```python
from build123d import *

# Parameters (mm, degrees)
SKETCH_1_W          = 120
SKETCH_1_H          = 94
SKETCH_1_R          = 37
EXTRUDE_2_DEPTH     = 4
SKETCH_2_W          = 15
SKETCH_2_H          = 74
CUT_EXTRUDE_1_DEPTH = 10
FILLET_1_R          = 8
FILLET_2_R          = 8
SKETCH_5_R          = 1.6
CUT_EXTRUDE_2_DEPTH = 10
SKETCH_6_W          = 10
SKETCH_6_H          = 43
EXTRUDE_3_DEPTH     = 4
FILLET_3_R          = 3.8
FILLET_4_R          = 15
SKETCH_7_R          = 1.6
CUT_EXTRUDE_3_DEPTH = 109.240473022
CUT_EXTRUDE_4_DEPTH = 10
FILLET_5_DEPTH      = 4
FILLET_6_R          = 5
MIRROR_1_DEPTH      = 4
SKETCH_10_R         = 1.6
CUT_EXTRUDE_6_DEPTH = 109.240473022


with BuildPart() as part:
    # 草图1 → 凸台-拉伸2 (new body)
    with BuildSketch(Plane(origin=(0, 0, 0), x_dir=(1, 0, 0), z_dir=(0, 1, 0))):
        Rectangle(SKETCH_1_W, SKETCH_1_H)
        with Locations(Location((0, 0, 0), (0, 0, 270))):
            Circle(SKETCH_1_R, mode=Mode.SUBTRACT)
    extrude(amount=EXTRUDE_2_DEPTH)

    # 草图2 → 切除-拉伸1 (cut)
    with BuildSketch(Plane(origin=(0, 4, 0), x_dir=(1, 0, 0), z_dir=(0, 1, 0))):
        with Locations((-52.5, 0)):
            Rectangle(SKETCH_2_W, SKETCH_2_H)
        with Locations((52.5, 0)):
            Rectangle(SKETCH_2_W, SKETCH_2_H)
    extrude(amount=-CUT_EXTRUDE_1_DEPTH, mode=Mode.SUBTRACT)

    # 圆角1
    fillet_1_edges = [part.edges().sort_by_distance(p)[0] for p in [
        (-45, 2, -37),
        (45, 2, -37),
    ]]
    fillet(fillet_1_edges, radius=FILLET_1_R)

    # 圆角2
    fillet_2_edges = [part.edges().sort_by_distance(p)[0] for p in [
        (-45, 2, 37),
        (45, 2, 37),
    ]]
    fillet(fillet_2_edges, radius=FILLET_2_R)

    # 草图5 → 切除-拉伸2 (cut)
    with BuildSketch(Plane(origin=(0, 4, 0), x_dir=(1, 0, 0), z_dir=(0, 1, 0))):
        with Locations(Location((-55, 42, 0), (0, 0, 270))):
            Circle(SKETCH_5_R)
        with Locations(Location((-55, -42, 0), (0, 0, 270))):
            Circle(SKETCH_5_R)
        with Locations(Location((55, -42, 0), (0, 0, 270))):
            Circle(SKETCH_5_R)
        with Locations(Location((55, 42, 0), (0, 0, 270))):
            Circle(SKETCH_5_R)
    extrude(amount=-CUT_EXTRUDE_2_DEPTH, mode=Mode.SUBTRACT)

    # 草图6 → 凸台-拉伸3 (add)
    with BuildSketch(Plane(origin=(0, 4, 0), x_dir=(1, 0, 0), z_dir=(0, 1, 0))):
        with Locations((-37.5, -68.5)):
            Rectangle(SKETCH_6_W, SKETCH_6_H)
        with Locations((37.5, -68.5)):
            Rectangle(SKETCH_6_W, SKETCH_6_H)
    extrude(amount=-EXTRUDE_3_DEPTH)

    # 圆角3
    fillet_3_edges = [part.edges().sort_by_distance(p)[0] for p in [
        (-42.5, 2, 47),
        (42.5, 2, 47),
    ]]
    fillet(fillet_3_edges, radius=FILLET_3_R)

    # 圆角4
    fillet_4_edges = [part.edges().sort_by_distance(p)[0] for p in [
        (-32.5, 2, 47),
        (32.5, 2, 47),
    ]]
    fillet(fillet_4_edges, radius=FILLET_4_R)

    # 草图7 → 切除-拉伸3 (cut, through all)
    with BuildSketch(Plane(origin=(0, 4, 0), x_dir=(1, 0, 0), z_dir=(0, 1, 0))):
        with Locations(Location((-20, 34.641016151, 0), (0, 0, 270))):
            Circle(SKETCH_7_R)
        with Locations(Location((20, 34.641016151, 0), (0, 0, 270))):
            Circle(SKETCH_7_R)
        with Locations(Location((40, 0, 0), (0, 0, 270))):
            Circle(SKETCH_7_R)
        with Locations(Location((20, -34.641016151, 0), (0, 0, 270))):
            Circle(SKETCH_7_R)
        with Locations(Location((-20, -34.641016151, 0), (0, 0, 270))):
            Circle(SKETCH_7_R)
        with Locations(Location((-40, 0, 0), (0, 0, 270))):
            Circle(SKETCH_7_R)
    extrude(amount=-CUT_EXTRUDE_3_DEPTH, mode=Mode.SUBTRACT)

    # 草图8 → 切除-拉伸4 (cut)
    with BuildSketch(Plane(origin=(0, 4, 0), x_dir=(1, 0, 0), z_dir=(0, 1, 0))):
        with BuildLine():
            Line((-20, 41.5), (-53, 41.5))
            ThreePointArc((-53, 41.5), (-42.247051947, 35.373704431), (-42.034221976, 22.999857308))
            Line((-42.034221976, 22.999857308), (-36.845014161, 20.160479446))
            ThreePointArc((-36.845014161, 20.160479446), (-31.047174279, 28.285561145), (-23.495769227, 34.813055431))
            ThreePointArc((-23.495769227, 34.813055431), (-22.413282259, 37.175985331), (-20, 38.141016151))
            Line((-20, 38.141016151), (-20, 41.5))
        make_face()
        with BuildLine():
            ThreePointArc((-24.974500131, -33.76794846), (-30.447809443, -28.929758038), (-35, -23.216373532))
            Line((-35, -23.216373532), (-35, -47.981599748))
            ThreePointArc((-35, -47.981599748), (-28.117207257, -42.250558092), (-19.540408864, -39.670596128))
            ThreePointArc((-19.540408864, -39.670596128), (-23.715698209, -38.061759575), (-24.974500131, -33.76794846))
        make_face()
    extrude(amount=-CUT_EXTRUDE_4_DEPTH, mode=Mode.SUBTRACT)

    # 圆角5: read off the stored shape, not the designer's step
    # 圆角5 outline → 圆角5 (add)
    with BuildSketch(Plane(origin=(0, 0, 0), x_dir=(1, 0, 0), z_dir=(0, 1, 0))):
        with BuildLine():
            ThreePointArc((-19.540408738, -39.670596116), (-22.017157734, -39.271240058), (-23.996197034, -37.729431281))
            ThreePointArc((-23.996197034, -37.729431281), (-23.660968385, -39.520217427), (-24.917103069, -40.839845755))
            ThreePointArc((-24.917103069, -40.839845755), (-22.264757976, -40.089668486), (-19.540408738, -39.670596116))
        make_face()
        with BuildLine():
            ThreePointArc((-25.820706479, -33.125384782), (-25.257029121, -33.817171884), (-25.050340682, -34.685262575))
            ThreePointArc((-25.050340682, -34.685262575), (-25.033361166, -34.224874204), (-24.974500131, -33.76794846))
            ThreePointArc((-24.974500131, -33.76794846), (-25.399635345, -33.449342659), (-25.820706479, -33.125384782))
        make_face()
        with BuildLine():
            ThreePointArc((-35, -47.981599748), (-33.451395129, -46.241873872), (-31.730675246, -44.672177642))
            ThreePointArc((-31.730675246, -44.672177642), (-33.854795441, -44.934725986), (-35, -43.12659857))
            Line((-35, -43.12659857), (-35, -47.981599748))
        make_face()
        with BuildLine():
            ThreePointArc((-35, -29.103264422), (-33.707106781, -27.232435728), (-31.5, -27.780388766))
            ThreePointArc((-31.5, -27.780388766), (-33.328217156, -25.55836343), (-35, -23.216373532))
            Line((-35, -23.216373532), (-35, -29.103264422))
        make_face()
        with BuildLine():
            Line((-20, 41.5), (-22, 41.5))
            ThreePointArc((-22, 41.5), (-20.633341947, 40.960221136), (-20.004377025, 39.632245767))
            ThreePointArc((-20.004377025, 39.632245767), (-20.386776912, 38.582327726), (-21.272727273, 37.901409577))
            ThreePointArc((-21.272727273, 37.901409577), (-20.647542667, 38.080592941), (-20, 38.141016151))
            Line((-20, 38.141016151), (-20, 41.5))
        make_face()
        with BuildLine():
            ThreePointArc((-44.379310345, 38.051724138), (-44.856953382, 40.242781353), (-43, 41.5))
            Line((-43, 41.5), (-53, 41.5))
            ThreePointArc((-53, 41.5), (-48.357616546, 40.605958636), (-44.379310345, 38.051724138))
        make_face()
        with BuildLine():
            ThreePointArc((-23.495769227, 34.813055431), (-23.462294071, 35.153382983), (-23.395766463, 35.488819274))
            ThreePointArc((-23.395766463, 35.488819274), (-23.686578053, 34.842467526), (-24.184558784, 34.338129192))
            ThreePointArc((-24.184558784, 34.338129192), (-23.841346618, 34.577307464), (-23.495769227, 34.813055431))
        make_face()
        with BuildLine():
            ThreePointArc((-35.890546019, 21.814415107), (-37.081603023, 20.921446591), (-38.55964247, 21.098672295))
            Line((-38.55964247, 21.098672295), (-36.845014161, 20.160479446))
            ThreePointArc((-36.845014161, 20.160479446), (-36.377181096, 20.992872494), (-35.890546019, 21.814415107))
        make_face()
    extrude(amount=FILLET_5_DEPTH)

    # 圆角6
    # the kernel refuses this fillet: 5 mm, written as the material it adds along each edge
    with BuildSketch(Plane(origin=(-42.034221976, 4, -22.999857308), x_dir=(0.8772622419285397, 0, 0.48001141537104314), z_dir=(0, -1, 0))) as fillet_6_piece_1:
        with BuildLine():
            CenterArc((4.273425175, -4.99021121), FILLET_6_R, 93.585816178, 69.846074329)
            ThreePointArc((-0.518982018, -3.564436578), (-0.130425942, -1.801010165), (0, 0))
            Line((0, 0), (3.960707916, 0))
        make_face()
    extrude(amount=4)

    # 镜向1: read off the stored shape, not the designer's step
    # 镜向1 outline → 镜向1 (cut)
    with BuildSketch(Plane(origin=(0, 0, 0), x_dir=(1, 0, 0), z_dir=(0, 1, 0))):
        with BuildLine():
            ThreePointArc((31.5, -27.780388766), (28.78468505, -30.584994795), (25.820706479, -33.125384782))
            ThreePointArc((25.820706479, -33.125384782), (25.257029121, -33.817171884), (25.050340682, -34.685262575))
            ThreePointArc((25.050340682, -34.685262575), (24.77249431, -36.293649447), (23.996197034, -37.729431281))
            ThreePointArc((23.996197034, -37.729431281), (23.660968385, -39.520217427), (24.917103069, -40.839845755))
            ThreePointArc((24.917103069, -40.839845755), (28.492191247, -42.456784369), (31.730675246, -44.672177642))
            ThreePointArc((31.730675246, -44.672177642), (33.854795441, -44.934725986), (35, -43.12659857))
            Line((35, -43.12659857), (35, -29.103264422))
            ThreePointArc((35, -29.103264422), (33.707106781, -27.232435728), (31.5, -27.780388766))
        make_face()
        with BuildLine():
            ThreePointArc((24.184558784, 34.338129192), (30.683308295, 28.679863879), (35.890546019, 21.814415107))
            ThreePointArc((35.890546019, 21.814415107), (37.081603023, 20.921446591), (38.55964247, 21.098672295))
            ThreePointArc((38.55964247, 21.098672295), (40.499095767, 23.388308225), (40.778535058, 26.375920225))
            ThreePointArc((40.778535058, 26.375920225), (41.05512866, 32.683754699), (44.379310345, 38.051724138))
            ThreePointArc((44.379310345, 38.051724138), (44.856953382, 40.242781353), (43, 41.5))
            Line((43, 41.5), (22, 41.5))
            ThreePointArc((22, 41.5), (20.633341947, 40.960221136), (20.004377025, 39.632245767))
            ThreePointArc((20.004377025, 39.632245767), (20.386776912, 38.582327726), (21.272727273, 37.901409577))
            ThreePointArc((21.272727273, 37.901409577), (22.627519064, 36.953189062), (23.395766462, 35.488819274))
            ThreePointArc((23.395766462, 35.488819274), (23.686578053, 34.842467526), (24.184558784, 34.338129192))
        make_face()
    extrude(amount=MIRROR_1_DEPTH, mode=Mode.SUBTRACT)

    # 草图10 → 切除-拉伸6 (cut, through all)
    with BuildSketch(Plane(origin=(0, 4, 0), x_dir=(1, 0, 0), z_dir=(0, 1, 0))):
        with Locations(Location((-39.5, -85, 0), (0, 0, 270))):
            Circle(SKETCH_10_R)
        with Locations(Location((-39.5, -65, 0), (0, 0, 270))):
            Circle(SKETCH_10_R)
        with Locations(Location((39.5, -65, 0), (0, 0, 90))):
            Circle(SKETCH_10_R)
        with Locations(Location((39.5, -85, 0), (0, 0, 90))):
            Circle(SKETCH_10_R)
    extrude(amount=-CUT_EXTRUDE_6_DEPTH, mode=Mode.SUBTRACT)


solid = part.part
```
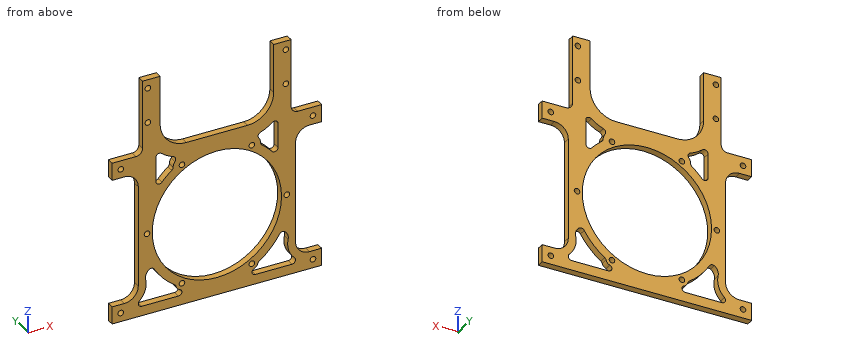
Read the model definition and answer for the solid it produces. Units are mm, in the model's axes. Round coordinates to 2 decimals unless told otherwise and drop trailing zeros. Write each loop counter-clockwise with the first axis right and the second up, starting at its lowest first coordinate (ties: lowest second). Pieces come first, ordered by that corner, then holes. Notation, with made-up numbers: (-19.5, 49.25) - (-12.5, 49.25) arc R7 cw to (-12.5, 60.25) - close; hole circle Ø7 at (79.25, -22). An arc over 180 degrees is marked (long way). Use CSV: the item, a comma, the result in double quotes.
Q1. Each of these flat-tipped pins is pushed along its axis until it touches: pin 1 Ø2 at (x, y) = (51, 1) entering from +Z; pin 2 Ø2 at (y, z) = (3, 75) entering from -X. Where does it stop, or does it pass through?
Values:
pin 1,"stops at z = 47"
pin 2,"stops at x = -42.5"
Q2. Straight lines are drawn through the part: line 1 along X through (y, z) = (1.25, -42); line 2 along X through (y, z) = (2.85, 85); line 3 along X through (y, z) = (1.85, 71). For each, find the intervals that lie inside material, in ascending order.
Values:
line 1,"x = -60 to -56.6, -53.4 to 53.4, 56.6 to 60"
line 2,"x = -42.5 to -41.1, -37.9 to -32.5, 32.5 to 37.9, 41.1 to 42.5"
line 3,"x = -42.5 to -32.5, 32.5 to 42.5"
Q3. Find section C-C, the plane y = 2.9. Count the separate pieces of the cut face and the enclosed holes in it, then the cut area to 3 significant figures.
Values:
separate pieces,"1"
enclosed holes,"19"
area,"4,820 mm²"
Q4. Find section B-B, the plane z = 48.5. Write down the section's boundary in (x, y).
Values:
outline,"(-43.28, 0) - (-24.04, 0) - (-24.04, 4) - (-43.28, 4) - close; (24.04, 0) - (43.28, 0) - (43.28, 4) - (24.04, 4) - close"
Q5. Find section A-A, the plane x = 48. Write down the section's boundary in (y, z) (3 decimals), then the cut area to 3 significant figures.
Values:
outline,"(0, -47) - (4, -47) - (4, -35.245) - (0, -35.245) - close; (0, 35.245) - (4, 35.245) - (4, 47) - (0, 47) - close"
area,"94.0 mm²"
